Can you work these out from the drawing? Everything is in mm from the part's minimum corner. A direction names the side the tool comes from. Round coordinates to 2 decimals unless told otherwise and drop trailing zeros. Write each loop counter-clockwise with the first axis right and the second up, starting at its lowest first coordinate (ties: lowest second). Pieces come first, ordered by that corner, then holes. Notation, with made-up numbers: (21.5, 54.5) - (76.5, 54.5) arc R32 cw to (76.5, 80.5) - close; hole circle Ø2 at (-2.75, 30.25). An arc over 180 degrees is marked (long way). One line per item, written item: value. Start each with the question number.
Item 1: Imagine slicing it at D-D, the plane x = 9.5. Please give me the cut outline in (y, z).
Item 2: Imagine slicing it at A-A, the plane z = 10. Please give me the cut outline in (x, y), then the cut area to 3 significant figures.
Item 3: For the marked faces 1 and 2, which set-ups out of +Z, -Z, +X, -X, +Y, -Y let a thin tool reach every point of the face, with its end or its side?
Item 4: If I drill on line 1 (X direction, y = 1.05, z = 10); line 2 (Y direction, x = 1, z = 14); line 3 (X direction, y = 2.3, z = 12.5), over which ranges is the centre line in solid material (lowest first)?
Item 5: Imagine slicing it at B-B, the plane x = 2.5. Please give me the cut outline in (y, z), then the cut area to 3 significant figures.
Item 6: For P1, Ø2, axis at x = 5, z = 4.5, coming from the +Y side; P2, Ø3, axis at y = 0.5, z = 13, coming from the -X side; P3, Ø2, axis at x = 14.5, y = 4, coming from the -Z side, each with a flat end and sliding along its axis, tell me the tip position at first contact or that it passes through.
Item 7: Thinking about a two-plate mould opening in X: for the marked faces 3, 4 and 5, which applies, released by +X, released by -X, zero draft, split by the parting line, or undercut?
Item 8: Imagine slicing it at C-C, the plane z = 2.5. Please give me the cut outline in (x, y).
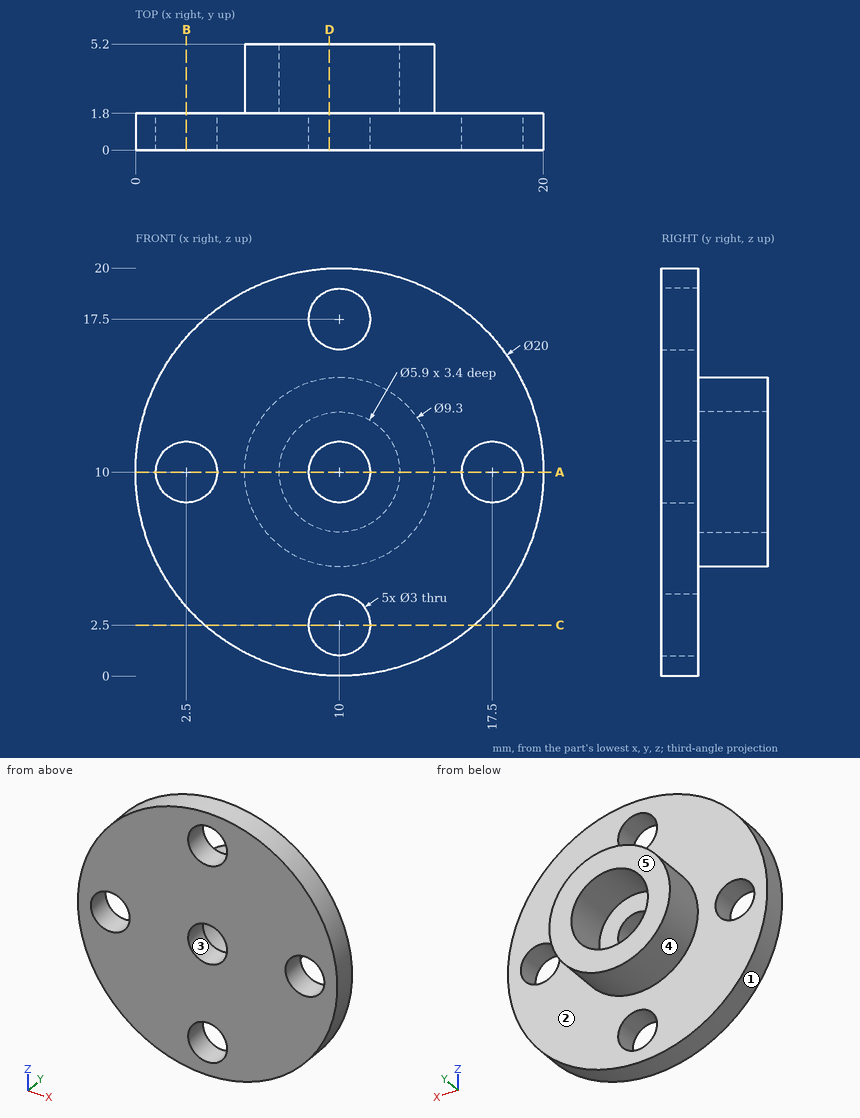
Values follow:
1. outline: (0, 0.01) - (1.8, 0.01) - (1.8, 1.09) - (0, 1.09) - close; (0, 3.91) - (1.8, 3.91) - (1.8, 5.38) - (5.2, 5.38) - (5.2, 7.09) - (1.8, 7.09) - (1.8, 8.59) - (0, 8.59) - close; (0, 11.41) - (1.8, 11.41) - (1.8, 12.91) - (5.2, 12.91) - (5.2, 14.62) - (1.8, 14.62) - (1.8, 16.09) - (0, 16.09) - close; (0, 18.91) - (1.8, 18.91) - (1.8, 19.99) - (0, 19.99) - close
2. outline: (0, 0) - (1, 0) - (1, 1.8) - (0, 1.8) - close; (4, 0) - (8.5, 0) - (8.5, 1.8) - (7.05, 1.8) - (7.05, 5.2) - (5.35, 5.2) - (5.35, 1.8) - (4, 1.8) - close; (11.5, 0) - (16, 0) - (16, 1.8) - (14.65, 1.8) - (14.65, 5.2) - (12.95, 5.2) - (12.95, 1.8) - (11.5, 1.8) - close; (19, 0) - (20, 0) - (20, 1.8) - (19, 1.8) - close
2. area: 31.4 mm^2
3. face 1: +Y, -Y
3. face 2: +Y
4. line 1: x = 0 to 1, 4 to 8.5, 11.5 to 16, 19 to 20
4. line 2: y = 0 to 1.8
4. line 3: x = 6.08 to 8.43, 11.57 to 13.92
5. outline: (0, 3.39) - (1.8, 3.39) - (1.8, 8.5) - (0, 8.5) - close; (0, 11.5) - (1.8, 11.5) - (1.8, 16.61) - (0, 16.61) - close
5. area: 18.4 mm^2
6. P1: stops at y = 1.8
6. P2: stops at x = 0.11
6. P3: stops at z = 6.94
7. face 3: undercut
7. face 4: split by the parting line
7. face 5: zero draft
8. outline: (3.39, 0) - (8.5, 0) - (8.5, 1.8) - (3.39, 1.8) - close; (11.5, 0) - (16.61, 0) - (16.61, 1.8) - (11.5, 1.8) - close
